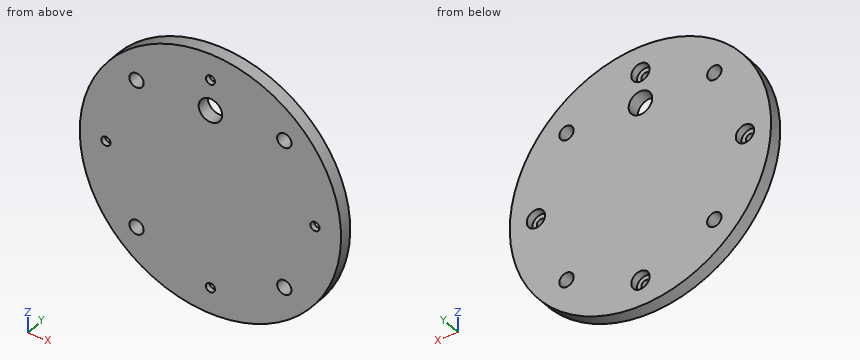
from build123d import *

# Parameters (mm, degrees)
SKETCH_1_R          = 50
EXTRUDE_1_DEPTH     = 5
SKETCH_2_R          = 1.75
CUT_EXTRUDE_1_DEPTH = 12
SKETCH_3_R          = 3.5
CUT_EXTRUDE_2_DEPTH = 3
SKETCH_4_R          = 2.75
CUT_EXTRUDE_3_DEPTH = 24
SKETCH_5_R          = 4.5
CUT_EXTRUDE_4_DEPTH = 16


with BuildPart() as part:
    # 草图1 → 凸台-拉伸1 (new body)
    with BuildSketch(Plane(origin=(0, 0, 0), x_dir=(1, 0, 0), z_dir=(0, 1, 0))):
        with Locations(Location((0, 0, 0), (0, 0, 270))):
            Circle(SKETCH_1_R)
    extrude(amount=EXTRUDE_1_DEPTH)

    # 草图2 → 切除-拉伸1 (cut)
    with BuildSketch(Plane(origin=(0, 5, 0), x_dir=(1, 0, 0), z_dir=(0, 1, 0))):
        with Locations(Location((0, 40, 0), (0, 0, 270))):
            Circle(SKETCH_2_R)
        with Locations(Location((40, 0, 0), (0, 0, 270))):
            Circle(SKETCH_2_R)
        with Locations(Location((0, -40, 0), (0, 0, 270))):
            Circle(SKETCH_2_R)
        with Locations(Location((-40, 0, 0), (0, 0, 270))):
            Circle(SKETCH_2_R)
    extrude(amount=-CUT_EXTRUDE_1_DEPTH, mode=Mode.SUBTRACT)

    # 草图3 → 切除-拉伸2 (cut)
    with BuildSketch(Plane(origin=(0, 5, 0), x_dir=(1, 0, 0), z_dir=(0, 1, 0))):
        with Locations(Location((0, 40, 0), (0, 0, 270))):
            Circle(SKETCH_3_R)
        with Locations(Location((40, 0, 0), (0, 0, 270))):
            Circle(SKETCH_3_R)
        with Locations(Location((0, -40, 0), (0, 0, 270))):
            Circle(SKETCH_3_R)
        with Locations(Location((-40, 0, 0), (0, 0, 270))):
            Circle(SKETCH_3_R)
    extrude(amount=-CUT_EXTRUDE_2_DEPTH, mode=Mode.SUBTRACT)

    # 草图4 → 切除-拉伸3 (cut)
    with BuildSketch(Plane(origin=(0, 5, 0), x_dir=(1, 0, 0), z_dir=(0, 1, 0))):
        with Locations(Location((28.284271247, 28.284271247, 0), (0, 0, 270))):
            Circle(SKETCH_4_R)
        with Locations(Location((28.284271247, -28.284271247, 0), (0, 0, 270))):
            Circle(SKETCH_4_R)
        with Locations(Location((-28.284271247, -28.284271247, 0), (0, 0, 270))):
            Circle(SKETCH_4_R)
        with Locations(Location((-28.284271247, 28.284271247, 0), (0, 0, 270))):
            Circle(SKETCH_4_R)
    extrude(amount=-CUT_EXTRUDE_3_DEPTH, mode=Mode.SUBTRACT)

    # 草图5 → 切除-拉伸4 (cut)
    with BuildSketch(Plane(origin=(0, 5, 0), x_dir=(1, 0, 0), z_dir=(0, 1, 0))):
        with Locations(Location((0, -28.284271247, 0), (0, 0, 270))):
            Circle(SKETCH_5_R)
    extrude(amount=-CUT_EXTRUDE_4_DEPTH, mode=Mode.SUBTRACT)


solid = part.part
Read the model definition and answer for the solid it produces. Units are mm, in the model's axes. Round coordinates to 2 decimals unless told otherwise and drop trailing zeros. Loops run counter-clockwise (first coordinate to the right, second up) from the corner with the lowest first, then second, coordinate; pieces in that order, holes last.
Q1. Section C-C on z = 28.5 is taken. Write down the section's boundary in (x, y), and give its area (3 significant figures).
Q2. Section B-B on x = -40 is taken. Write down the section's boundary in (y, z).
Q3. Consider probe 1 along X at (y, z) = (1.3, 0); probe 2 along X at (y, z) = (4.3, 0); probe 3 along Z at (x, y) = (-28, 3.7). Determine where each line is inside the solid, lowest interval first.
Q4. Section D-D on z = -40 is taken. Write down the section's boundary in (x, y), and give its area (3 significant figures).
Q5. Each of these flat-tipped pins is pushed along its axis until it touches: pin 1 (1 mm diameter, centred on x = 37, y = 4, fed in from -Z); pin 2 (4.5 mm diameter, centred on x = -28.28, z = 28.28, fed in from -Y) (1 decimal); pin 3 (11.5 mm diameter, centred on x = 0, z = 28.28, fed in from +Y); pin 4 (2 mm diameter, centred on x = 1, z = -39, fed in from +Y). Where does it stop, or does it pass through?
Q6. Section A-A on z = 0 is taken. Write down the section's boundary in (x, y), and give its area (3 significant figures).
Output:
1. outline: (-41.08, 0) - (-31.03, 0) - (-31.03, 5) - (-41.08, 5) - close; (-25.54, 0) - (-4.49, 0) - (-4.49, 5) - (-25.54, 5) - close; (4.49, 0) - (25.54, 0) - (25.54, 5) - (4.49, 5) - close; (31.03, 0) - (41.08, 0) - (41.08, 5) - (31.03, 5) - close
1. area: 311 mm2
2. outline: (0, -30) - (5, -30) - (5, -3.5) - (2, -3.5) - (2, -1.75) - (0, -1.75) - close; (0, 1.75) - (2, 1.75) - (2, 3.5) - (5, 3.5) - (5, 30) - (0, 30) - close
3. probe 1: x = -50 to -41.75, -38.25 to 38.25, 41.75 to 50
3. probe 2: x = -50 to -43.5, -36.5 to 36.5, 43.5 to 50
3. probe 3: z = -41.42 to -31.02, -25.55 to 25.55, 31.02 to 41.42
4. outline: (-30, 0) - (-1.75, 0) - (-1.75, 2) - (-3.5, 2) - (-3.5, 5) - (-30, 5) - close; (1.75, 0) - (30, 0) - (30, 5) - (3.5, 5) - (3.5, 2) - (1.75, 2) - close
4. area: 272 mm2
5. pin 1: stops at z = -34.17
5. pin 2: passes through
5. pin 3: stops at y = 5
5. pin 4: stops at y = 2
6. outline: (-50, 0) - (-41.75, 0) - (-41.75, 2) - (-43.5, 2) - (-43.5, 5) - (-50, 5) - close; (-38.25, 0) - (38.25, 0) - (38.25, 2) - (36.5, 2) - (36.5, 5) - (-36.5, 5) - (-36.5, 2) - (-38.25, 2) - close; (41.75, 0) - (50, 0) - (50, 5) - (43.5, 5) - (43.5, 2) - (41.75, 2) - close
6. area: 444 mm2
